Verification items for the finished model (mm, model axes). A direction names the side the tool comes from. Give positions to 0.01 mm unless a question says otherwise; leave off trailing zeros. Write each loop counter-clockwise with the first axis right and the second up, starting at its lowest first coordinate (ties: lowest second). Pieces come first, ordered by that corner, then holes. Notation, with made-up numbers: M 7,14.25 L 25,14.25 A28 cw 25,41.25 Z; hole C 8,89 d8. An arc over 180 degrees is marked long. Answer as a JSON object with one key per item and string values.
```python
from build123d import *

# Parameters (mm, degrees)
SKETCH1_R               = 25
BOSS_EXTRUDE1_DEPTH     = 30
SKETCH2_W               = 1.27
SKETCH2_H               = 1.27
SKETCH10_R              = 20
CUT_EXTRUDE1_DEPTH      = 25
CUT_EXTRUDE2_DEPTH      = 47.368092477
CUT_EXTRUDE2_DEPTH_BACK = 47.368092477
CUT_EXTRUDE3_DEPTH      = 47.368092477
CUT_EXTRUDE3_DEPTH_BACK = 47.368092477
SKETCH12_R              = 2.5


with BuildPart() as part:
    # Sketch1 → Boss-Extrude1 (new body)
    with BuildSketch(Plane(origin=(0, 0, 0), x_dir=(1, 0, 0), z_dir=(0, 1, 0))):
        with Locations(Location((0, 0, 0), (0, 0, 270))):
            Circle(SKETCH1_R)
    extrude(amount=BOSS_EXTRUDE1_DEPTH)

    # Sketch2 → Cut-Revolve1 (revolve, cut)
    with BuildSketch(Plane.XY, mode=Mode.PRIVATE) as cut_revolve1_sk:
        with Locations((24.365, 1.905)):
            Rectangle(SKETCH2_W, SKETCH2_H)
        with Locations((24.365, 4.445)):
            Rectangle(SKETCH2_W, SKETCH2_H)
        with Locations((24.365, 6.985)):
            Rectangle(SKETCH2_W, SKETCH2_H)
    revolve(cut_revolve1_sk.sketch.rotate(Axis((0, 0, 0), (0, 1, 0)), 90), axis=Axis((0, 0, 0), (0, 1, 0)), mode=Mode.SUBTRACT)

    # Sketch10 → Cut-Extrude1 (cut)
    with BuildSketch(Plane(origin=(0, 30, 0), x_dir=(1, 0, 0), z_dir=(0, 1, 0))):
        with Locations(Location((0, 0, 0), (0, 0, 270))):
            Circle(SKETCH10_R)
    extrude(amount=-CUT_EXTRUDE1_DEPTH, mode=Mode.SUBTRACT)

    # Sketch11 → Cut-Extrude2 (cut, two sides: drawn at the far end of the back side and taken through both)
    with BuildSketch(Plane(origin=(0, 0, 0), x_dir=(0, 0, -1), z_dir=(1, 0, 0)).offset(-CUT_EXTRUDE2_DEPTH_BACK)):
        Polygon((0, 16.523537724), (6.878930104, 16.523537724), (14.594122298, 30), (-14.540169905, 30), (-7.36450164, 16.523537724), align=None)
    extrude(amount=CUT_EXTRUDE2_DEPTH + CUT_EXTRUDE2_DEPTH_BACK, mode=Mode.SUBTRACT)

    # Sketch12 → Cut-Extrude3 (cut, two sides: drawn at the far end of the back side and taken through both)
    with BuildSketch(Plane.XY.offset(-CUT_EXTRUDE3_DEPTH_BACK)):
        with Locations((0, 18.210167382)):
            Circle(SKETCH12_R)
    extrude(amount=CUT_EXTRUDE3_DEPTH + CUT_EXTRUDE3_DEPTH_BACK, mode=Mode.SUBTRACT)


solid = part.part
```
1) Go/stop test with flat-tipped pins: pin 1 (5 mm diameter, centred on y = 6.5, z = 2, fed in from +X); pin 2 (15 mm diameter, centred on x = 9.5, z = -0.5, fed in from +Y); pin 3 (25 mm diameter, centred on x = -11, z = 7, fed in from -Y); pin 4 (3 mm diameter, centred on x = 0, y = 18.21, fed in from +Z). Record where each tip stops, or that it passes through.
Completed:
{"pin 1": "stops at x = 25", "pin 2": "stops at y = 5", "pin 3": "stops at y = 0", "pin 4": "passes through"}
2) Section check A-A on y = 25. Record the boundary of the cut face in (x, z), and give its area (3 significant figures).
Completed:
{"outline": "M -22.08,-11.73 A25 ccw 22.08,-11.73 L 16.2,-11.73 A20 cw -16.2,-11.73 Z; M -22,11.88 L -16.09,11.88 A20 cw 16.09,11.88 L 22,11.88 A25 ccw Z", "area": "458 mm2"}
3) Access from +Z, -Z, +X, -X, +Y, -Y to the whole of each face (thin tool, end or side, straight path). Record for faces 1 (the face through (-19, 6.35, 15)), 2 (the face through (7.509, 0.626, 23.846)), 3 (the face through (19.869, 23.356, 11.003)).
Completed:
{"face 1": "none", "face 2": "+Y, -Y", "face 3": "+X, -X, +Y"}
4) Release check for a two-part mould opening along Z. For faces 4 (the face through (0, 5, 0)), 5 (the face through (-7.128, 4.454, -22.634)), 6 (the face through (-19, 5.08, 15)) record: pulls with the +Z half, pulls with the -Z half, needs draft (parallel to the pull), parting line crosses it, or undercut.
Completed:
{"face 4": "undercut", "face 5": "parting line crosses it", "face 6": "needs draft"}
5) Thickness scan on L1, parallel to Y at x = 0, z = 23.85; L2, parallel to Y at x = 0, z = -21.3; L3, parallel to Z at x = 0, y = 21. Record the ranges inside material, lowest first.
Completed:
{"L1": "y = 0 to 1.27, 2.54 to 3.81, 5.08 to 6.35, 7.62 to 15.71, 20.71 to 30", "L2": "y = 0 to 15.71, 20.71 to 30", "L3": "z = -25 to -20, 20 to 25"}
6) Section check C-C on y = 9.5. Record the boundary of the cut face in (x, z).
Completed:
{"outline": "C 0,0 d50; hole C 0,0 d40"}
